Design review of the part shown in the three views and the two pictorial views. Dimensions are in mm from the part's minimum x, y and z. Round coordinates to 2 decimals unless told otherwise and drop trailing zeros. Order: outer loops, then holes, each group sorted by start corner. A loop starts at its lowest first (then second) coordinate and runs counter-clockwise, first axis right, second up. Notation, with made-up numbers: M -14,29 L 33,29 A18 cw 33,41 Z; hole C 36.25,61.25 d1. An arc over 180 degrees is marked long. Write item = value, one per line. Start each with the question number.
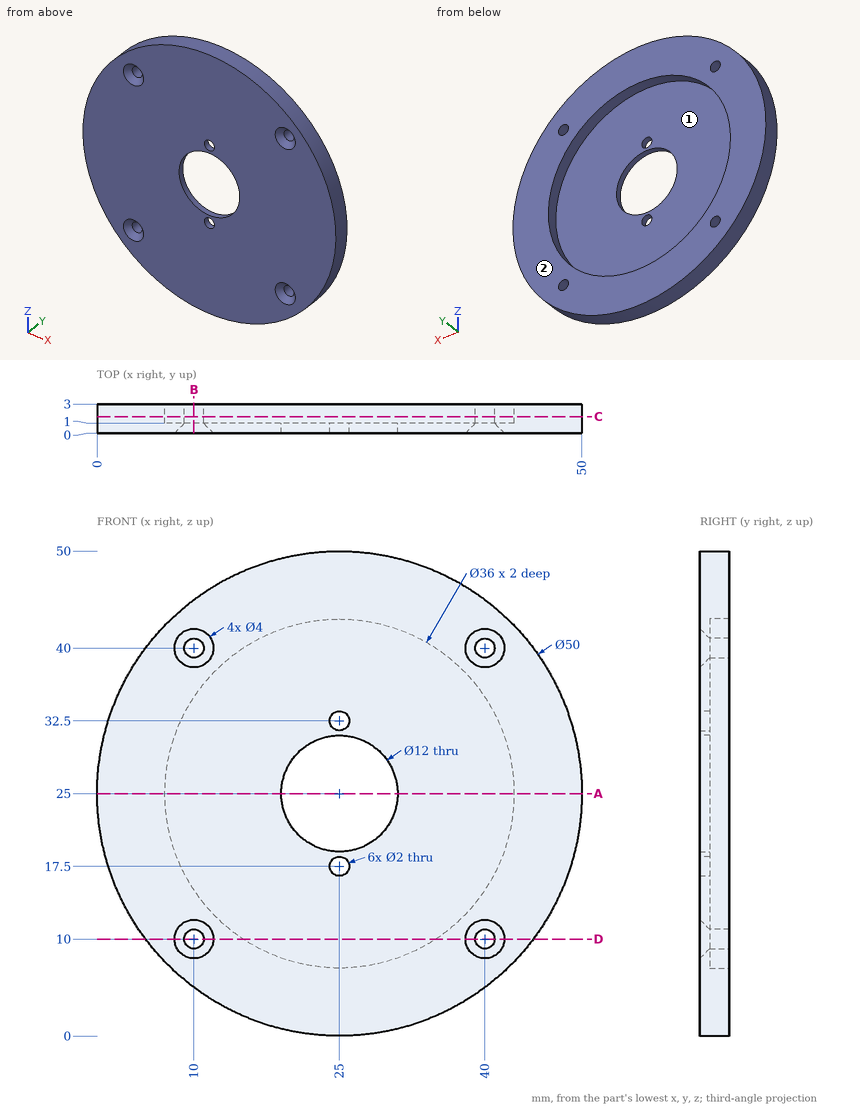
(1) Draft analysis for pull direction Z (two halves, no side actions). For the marked faces 1 and 2, state which applies: released by +Z, released by -Z, zero draft, split by the parting line, or undercut.
(2) We need section B-B, the plane x = 10. Write out the cut boundary in (y, z).
(3) Insertion check: pin 1 (1.8 mm diameter, centred on x = 10, z = 40, fed in from -Y); pin 2 (11 mm diameter, centred on x = 19.5, z = 18.5, fed in from +Y); pin 3 (1 mm diameter, centred on x = 21, y = 2, fed in from -Z); pin 4 (1 mm diameter, centred on y = 2.5, z = 18.5, fed in from +X). Each pin has a flat end and moves straight along its axis. Give the tip position at first contact, or say it passes through.
(4) For line 1 along X through (y, z) = (2.1, 25.5) (3 decimals); line 2 along X through (y, z) = (0.5, 25); line 3 along Y through (x, z) = (9, 27), list the stretches that pass through material, from the lowest coordinate up.
(5) We need section D-D, the plane z = 10. Write out the cut boundary in (x, y).
(6) We need section A-A, the plane z = 25. Write out the cut boundary in (x, y), then the cut area to 3 significant figures.
(7) We need section C-C, the plane y = 1.7. Write out the cut boundary in (x, z).
Values:
q1.face_1 = undercut
q1.face_2 = zero draft
q2.outline = M 0,5 L 3,5 L 3,9 L 1,9 L 0,8 Z; M 0,12 L 1,11 L 3,11 L 3,15.05 L 1,15.05 L 1,34.95 L 3,34.95 L 3,39 L 1,39 L 0,38 Z; M 0,42 L 1,41 L 3,41 L 3,45 L 0,45 Z
q3.pin_1 = through
q3.pin_2 = 1
q3.pin_3 = 0.25
q3.pin_4 = 49.27
q4.line_1 = 0.005 to 7.007, 42.993 to 49.995
q4.line_2 = 0 to 19, 31 to 50
q4.line_3 = 0 to 1
q5.outline = M 5,0 L 8,0 L 9,1 L 9,3 L 5,3 Z; M 11,1 L 12,0 L 38,0 L 39,1 L 39,3 L 34.95,3 L 34.95,1 L 15.05,1 L 15.05,3 L 11,3 Z; M 41,1 L 42,0 L 45,0 L 45,3 L 41,3 Z
q6.outline = M 0,0 L 19,0 L 19,1 L 7,1 L 7,3 L 0,3 Z; M 31,0 L 50,0 L 50,3 L 43,3 L 43,1 L 31,1 Z
q6.area = 66.0 mm²
q7.outline = C 25,25 d50; hole C 25,25 d36; hole C 10,10 d2; hole C 10,40 d2; hole C 40,10 d2; hole C 40,40 d2
